For this review, use the dimensioned drawing (mm, ordinates from the lowest corner) and the shaded views. Give positions to 0.01 mm unless a question says otherwise; leave off trailing zeros. Answer as CSV lines item,"result". Start each with the question number.
1. For line 1 along Z through (x, y) = (90.25, 0.75); line 2 along Z through (x, y) = (27, 1.3); line 3 along X through (y, z) = (1.75, 36), list the stretches that pass through material, from the lowest coordinate up.
2. We need section C-C, the plane y = 1.6. State how many separate pieces and enclosed holes the cut face has, and give its area (3 significant figures).
3. Clearance check with flat-ended pins moving along their axes: P1, Ø8, axis at x = 93.5, z = 73.5, coming from the -Y side; P2, Ø4, axis at x = 61.75, z = 110.375, coming from the -Y side; P3, Ø1, axis at x = 105.5, y = 0.5, coming from the -Z side. State where each tip first meets the part, or that it passes through.
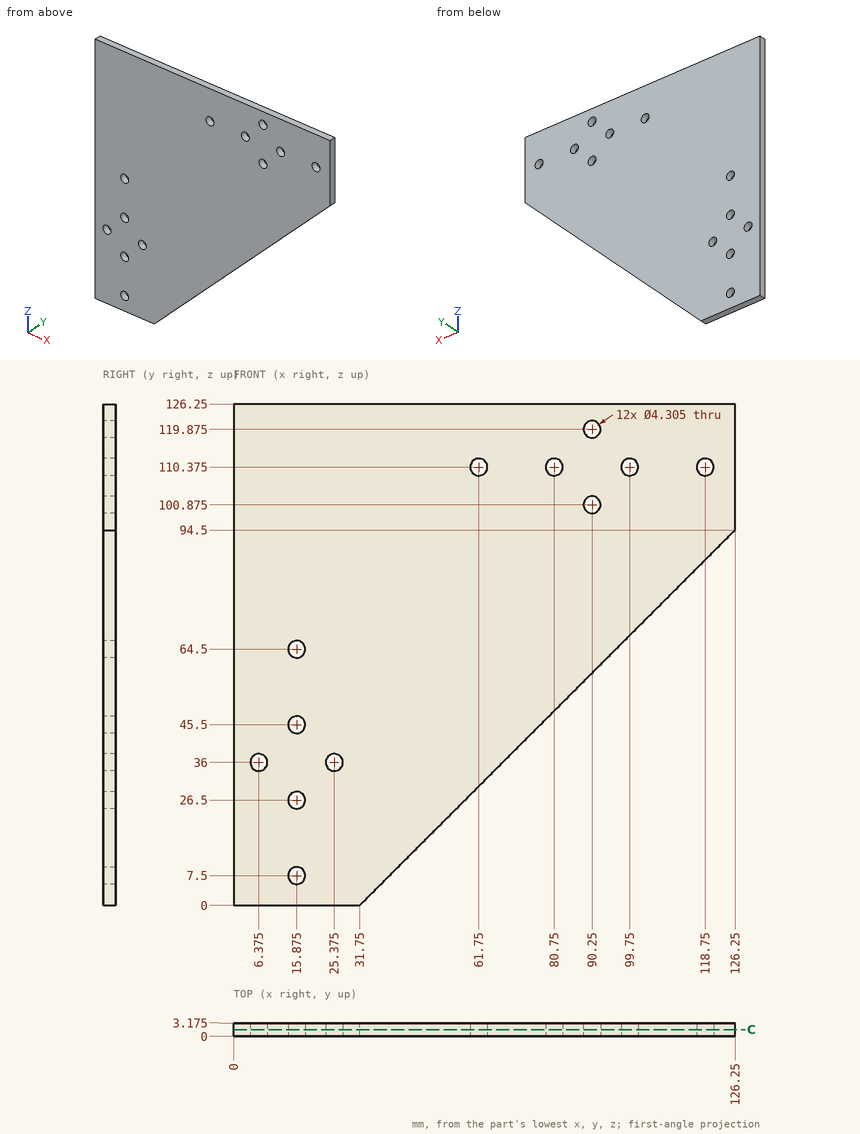
Result set:
1,line 1,"58.5 to 98.72, 103.03 to 117.72, 122.03 to 126.25"
1,line 2,"0 to 34.59, 37.41 to 126.25"
1,line 3,"0 to 4.22, 8.53 to 23.22, 27.53 to 67.75"
2,separate pieces,"1"
2,enclosed holes,"12"
2,area,"11,300 mm2"
3,P1,"y = 0"
3,P2,"through"
3,P3,"z = 73.25"
